Geometry: final body of the model. Coordinates: model frame, mm. Face numbers are marked on the shaded views. A direction names the side the tool comes from. Give positions to 0.01 mm unless a question says otherwise; leave off trailing zeros. Order: outer loops, then holes, each group sorted by start corner. A loop starts at its lowest first (then second) coordinate and runs counter-clockwise, first axis right, second up. Notation, with made-up numbers: (38, 70) -> (65, 70) arc R26 cw to (65, 105) -> close; hole circle Ø7 at (10.5, 25.5). An arc over 180 degrees is marked (long way). Answer in a Markdown table with one row per item. Add a question column.
Q1. Cut plane A-A on z = 7.5. Return the cut outline in (x, y).
Q2. Cut plane C-C on y = 0. Return the cut outline in (x, z).
Q3. Line query: line 1 along X through (y, z) = (0, 4.5); line 2 along X through (y, z) = (0, 0.65); line 3 along Y through (x, z) = (7.25, 6.75). Output: solid intervals per line, ascending. Write a range as from..to.
Q4. Set-up query: the marked faces 1, 2, 3, 4 and 5. Return all of +Z, -Z, +X, -X, +Y, -Y with unobstructed straight access to the full face (end or side cutting, diameter ignored); none if empty.
Q5. Cut plane B-B on x = 18.5. Return the cut outline in (y, z).
Q6. Cut plane D-D on z = 4.5. Return the cut outline in (x, y), and give its area (3 significant figures).
Q7. Contact query for flat-ended pins moving along their axis: P1, Ø0.8, axis at x = 16, z = 0.5, coming from the -Y side; P2, Ø1.5, axis at x = 2, z = 8.5, coming from the +Y side; P3, Ø6.5, axis at x = 6.5, z = 10, coming from the +Y side; P4, Ø1.8, axis at x = -7.25, y = 0, coming from the +Z side. Output: stop coordinate, or through.
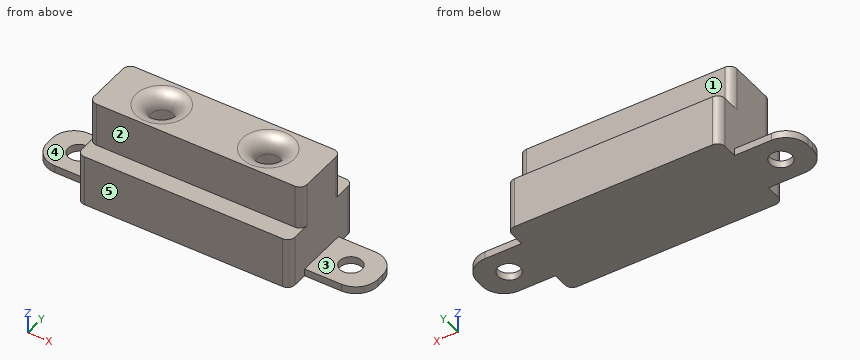
Autodesk Inventor part; units mm, degrees
ref_plane "YZ Plane" through (0, 0, 0) normal (1, 0, 0) x (0, 1, 0)
ref_plane "XZ Plane" through (0, 0, 0) normal (0, 1, 0) x (-1, 0, 0)
ref_plane "XY Plane" through (0, 0, 0) normal (0, 0, 1) x (1, 0, 0)
sketch "スケッチ1" plane through (0, 0, 0) normal (0, 0, 1) x (1, 0, 0)
  line L0 (-22.5, 6.5) -> (22.5, 6.5)
  line L1 (22.5, 6.5) -> (22.5, -6.5)
  line L2 (22.5, -6.5) -> (-22.5, -6.5)
  line L3 (-22.5, -6.5) -> (-22.5, 6.5)
  line L4 (-22.5, 6.5) -> (22.5, -6.5) construction
  line L5 (22.5, 6.5) -> (-22.5, -6.5) construction
  point P0 (0, 0)
  dimension "d0" = 45
  dimension "d1" = 13
extrude "押し出し1" add sketch "スケッチ1" along normal blind 1
sketch "スケッチ2" plane through (0, 0, 1) normal (0, 0, 1) x (1, 0, 0)
  line L0 (-14.5, 6.5) -> (14.5, 6.5)
  line L1 (14.5, 6.5) -> (14.5, -6.5)
  line L2 (14.5, -6.5) -> (-14.5, -6.5)
  line L3 (-14.5, -6.5) -> (-14.5, 6.5)
  line L4 (-14.5, 6.5) -> (14.5, -6.5) construction
  line L5 (14.5, 6.5) -> (-14.5, -6.5) construction
  point P0 (0, 0)
  dimension "d4" = 29
  dimension "d5" = 13
extrude "押し出し2" add sketch "スケッチ2" along normal blind 6
sketch "スケッチ4" plane through (0, 0, 7) normal (0, 0, 1) x (1, 0, 0)
  line L0 (-14.5, 4) -> (14.5, 4)
  line L1 (14.5, 4) -> (14.5, -4)
  line L2 (14.5, -4) -> (-14.5, -4)
  line L3 (-14.5, -4) -> (-14.5, 4)
  line L4 (-14.5, 4) -> (14.5, -4) construction
  line L5 (14.5, 4) -> (-14.5, -4) construction
  point P0 (0, 0)
  dimension "d8" = 29
  dimension "d9" = 8
extrude "押し出し3" add sketch "スケッチ4" along normal blind 6
sketch "スケッチ5" plane through (0, 0, 1) normal (0, 0, 1) x (1, 0, 0)
  point P0 (0, 0)
sketch "スケッチ6" plane through (0, 0, 1) normal (0, 0, 1) x (1, 0, 0)
  line L0 (22.5, 6.5) -> (14.5, 6.5)
  line L1 (14.5, 6.5) -> (14.5, 3.5)
  line L2 (14.5, 3.5) -> (22.5, 3.5)
  line L3 (22.5, 3.5) -> (22.5, 6.5)
  line L4 (22.5, -6.5) -> (14.5, -6.5)
  line L5 (14.5, -6.5) -> (14.5, -3.5)
  line L6 (14.5, -3.5) -> (22.5, -3.5)
  line L7 (22.5, -3.5) -> (22.5, -6.5)
  line L8 (-22.5, 6.5) -> (-14.5, 6.5)
  line L9 (-14.5, 6.5) -> (-14.5, 3.5)
  line L10 (-14.5, 3.5) -> (-22.5, 3.5)
  line L11 (-22.5, 3.5) -> (-22.5, 6.5)
  line L12 (-22.5, -6.5) -> (-14.5, -6.5)
  line L13 (-14.5, -6.5) -> (-14.5, -3.5)
  line L14 (-14.5, -3.5) -> (-22.5, -3.5)
  line L15 (-22.5, -3.5) -> (-22.5, -6.5)
  point P0 (0, 0)
  dimension "d12" = 8
  dimension "d13" = 3
  dimension "d14" = 8
  dimension "d15" = 3
  dimension "d16" = 8
  dimension "d17" = 3
  dimension "d18" = 8
  dimension "d19" = 3
extrude "押し出し4" cut sketch "スケッチ6" against normal blind 6
fillet "フィレット1" radius 3 4 edges at (22.5, 3.5, 0.5) (22.5, -3.5, 0.5) (-22.5, 3.5, 0.5) (-22.5, -3.5, 0.5)
sketch "スケッチ7" plane through (0, 0, 13) normal (0, 0, 1) x (1, 0, 0)
  point P0 (0, 0)
  point P1 (7.25, 0)
  point P2 (-7.25, 0)
  point P3 (-18.5, 0)
  point P4 (18.5, 0)
hole "穴1" at (7.25, 0, 13) at (-7.25, 0, 13) at (-18.5, 0, 13) at (18.5, 0, 13) direction (0, 0, -1) diameter 3 end through all
fillet "フィレット2" radius 2 2 edges at (-7.25, 1.5, 13) (7.25, 1.5, 13)
sketch "スケッチ8" plane through (0, 0, 0) normal (0, 0, -1) x (-1, 0, 0)
  line L0 (12.5, -3.5) -> (-12.5, -3.5)
  line L1 (-12.5, -3.5) -> (-12.5, 3.5)
  line L2 (-12.5, 3.5) -> (12.5, 3.5)
  line L3 (12.5, 3.5) -> (12.5, -3.5)
  line L4 (12.5, -3.5) -> (-12.5, 3.5) construction
  line L5 (-12.5, -3.5) -> (12.5, 3.5) construction
  point P0 (0, 0)
  dimension "d31" = 7
  dimension "d32" = 25
extrude "押し出し5" cut sketch "スケッチ8" against normal blind 2
sketch "スケッチ9" plane through (0, 0, 2) normal (0, 0, -1) x (-1, 0, 0)
  line L0 (12.5, -3.5) -> (-12.5, -3.5)
  line L1 (-12.5, -3.5) -> (-12.5, 3.5)
  line L2 (-12.5, 3.5) -> (12.5, 3.5)
  line L3 (12.5, 3.5) -> (12.5, -3.5)
  line L4 (12.5, -3.5) -> (-12.5, 3.5) construction
  line L5 (-12.5, -3.5) -> (12.5, 3.5) construction
  point P0 (0, 0)
  dimension "d35" = 25
  dimension "d36" = 7
extrude "押し出し6" add sketch "スケッチ9" along normal blind 2
fillet "フィレット3" radius 1 8 edges at (14.5, 4, 10) (14.5, 6.5, 3.5) (14.5, -4, 10) (14.5, -6.5, 3.5) (-14.5, 6.5, 3.5) (-14.5, 4, 10) (-14.5, -4, 10) (-14.5, -6.5, 3.5)
properties part number "PSDセンサ" material "アセタール樹脂、黒"
Completed:
| question | item | result |
|---|---|---|
| 1 | outline | (-14.5, -3) arc R1 ccw to (-13.5, -4) -> (13.5, -4) arc R1 ccw to (14.5, -3) -> (14.5, 3) arc R1 ccw to (13.5, 4) -> (-13.5, 4) arc R1 ccw to (-14.5, 3) -> close; hole circle Ø3 at (-7.25, 0); hole circle Ø3 at (7.25, 0) |
| 2 | outline | (-22.5, 0) -> (-20, 0) -> (-20, 1) -> (-22.5, 1) -> close; (-17, 0) -> (17, 0) -> (17, 1) -> (14.5, 1) -> (14.5, 13) -> (10.75, 13) arc R2 ccw to (8.75, 11) -> (8.75, 2) -> (5.75, 2) -> (5.75, 11) arc R2 ccw to (3.75, 13) -> (-3.75, 13) arc R2 ccw to (-5.75, 11) -> (-5.75, 2) -> (-8.75, 2) -> (-8.75, 11) arc R2 ccw to (-10.75, 13) -> (-14.5, 13) -> (-14.5, 1) -> (-17, 1) -> close; (20, 0) -> (22.5, 0) -> (22.5, 1) -> (20, 1) -> close |
| 3 | line 1 | x = -14.5..-8.75, -5.75..5.75, 8.75..14.5 |
| 3 | line 2 | x = -22.5..-20, -17..17, 20..22.5 |
| 3 | line 3 | y = -6.5..-1.5, 1.5..6.5 |
| 4 | face 1 | +Z, +X, -X, +Y |
| 4 | face 2 | +Z, +X, -X, -Y |
| 4 | face 3 | +Z, +X, +Y, -Y |
| 4 | face 4 | +Z, -X, +Y, -Y |
| 4 | face 5 | +Z, -Z, +X, -X, -Y |
| 5 | outline | (-3.5, 0) -> (-1.5, 0) -> (-1.5, 1) -> (-3.5, 1) -> close; (1.5, 0) -> (3.5, 0) -> (3.5, 1) -> (1.5, 1) -> close |
| 6 | outline | (-14.5, -5.5) arc R1 ccw to (-13.5, -6.5) -> (13.5, -6.5) arc R1 ccw to (14.5, -5.5) -> (14.5, 5.5) arc R1 ccw to (13.5, 6.5) -> (-13.5, 6.5) arc R1 ccw to (-14.5, 5.5) -> close; hole circle Ø3 at (-7.25, 0); hole circle Ø3 at (7.25, 0) |
| 6 | area | 362 mm² |
| 7 | P1 | stops at y = -3.5 |
| 7 | P2 | stops at y = 4 |
| 7 | P3 | stops at y = 6.5 |
| 7 | P4 | stops at z = 2 |
